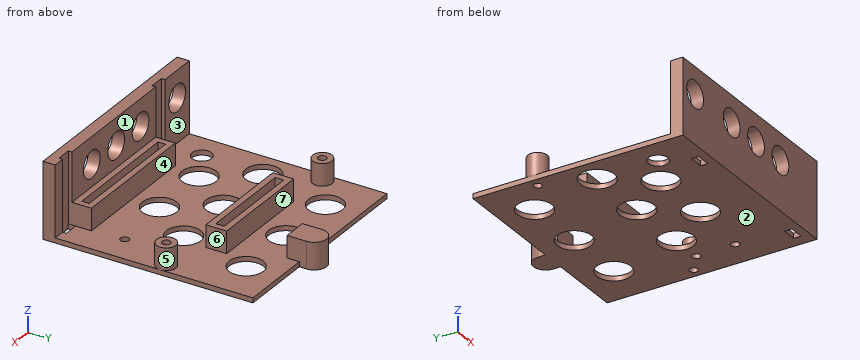
```python
from build123d import *

# Parameters (mm, degrees)
PAD_DEPTH       = 2
SKETCH001_W     = 50
SKETCH001_H     = 3
SKETCH001_W_2   = 44
SKETCH001_H_2   = 8.5
SKETCH001_W_3   = 39
SKETCH001_H_3   = 3.5
SKETCH001_R     = 4
PAD001_DEPTH    = 9
SKETCH003_R     = 1.75
SKETCH003_R_2   = 7
SKETCH003_R_3   = 4
SKETCH003_W     = 6
SKETCH003_H     = 3
POCKET_DEPTH    = 5
PAD002_DEPTH    = 20
SKETCH006_R     = 5.5
POCKET001_DEPTH = 5
SKETCH004_R     = 1.7
POCKET002_DEPTH = 11


with BuildPart() as part:
    # Sketch → Pad (new body)
    with BuildSketch(Plane.XY):
        with BuildLine():
            Line((0, 0), (0, 86))
            Line((0, 86), (47.5, 86))
            Line((47.5, 86), (47.5, 89))
            ThreePointArc((57.5, 89), (52.5, 94), (47.5, 89))
            Line((57.5, 89), (57.5, 86))
            Line((57.5, 86), (88, 86))
            Line((88, 86), (88, 0))
            Line((88, 0), (0, 0))
        make_face()
    extrude(amount=PAD_DEPTH)

    # Sketch001 → Pad001 (new body)
    with BuildSketch(Plane.XY.offset(2)):
        Polygon((0, 0), (0, 5), (15.9, 5), (15.9, 3.5), (22, 3.5), (22, 13), (77, 13), (77, 3.5), (83.1, 3.5), (83.1, 5), (88, 5), (88, 0), align=None)
        with Locations((49.5, 9)):
            Rectangle(SKETCH001_W, SKETCH001_H, mode=Mode.SUBTRACT)
        with Locations((44, 57.25)):
            Rectangle(SKETCH001_W_2, SKETCH001_H_2)
        with Locations((44, 57.25)):
            Rectangle(SKETCH001_W_3, SKETCH001_H_3, mode=Mode.SUBTRACT)
        with BuildLine():
            Line((47.5, 89), (47.5, 81))
            Line((47.5, 81), (57.5, 81))
            Line((57.5, 81), (57.5, 89))
            ThreePointArc((57.5, 89), (52.5, 94), (47.5, 89))
        make_face()
        with Locations((4, 62)):
            Circle(SKETCH001_R)
        with Locations((84, 48)):
            Circle(SKETCH001_R)
    extrude(amount=PAD001_DEPTH)

    # Sketch003 → Pocket (cut)
    with BuildSketch(Plane.XY.offset(2)):
        with Locations((76, 42)):
            Circle(SKETCH003_R)
        with Locations((76, 26)):
            Circle(SKETCH003_R)
        with Locations((37, 42)):
            Circle(SKETCH003_R_2)
        with Locations((24, 24)):
            Circle(SKETCH003_R_2)
        with Locations((63, 42)):
            Circle(SKETCH003_R_2)
        with Locations((50, 24)):
            Circle(SKETCH003_R_2)
        with Locations((70, 72)):
            Circle(SKETCH003_R_2)
        with Locations((44, 72)):
            Circle(SKETCH003_R_2)
        with Locations((18, 72)):
            Circle(SKETCH003_R_2)
        with Locations((11, 42)):
            Circle(SKETCH003_R_2)
        with Locations((11, 17)):
            Circle(SKETCH003_R_3)
        with Locations((80.1, 5)):
            Rectangle(SKETCH003_W, SKETCH003_H)
        with Locations((18.9, 5)):
            Rectangle(SKETCH003_W, SKETCH003_H)
    extrude(amount=-POCKET_DEPTH, mode=Mode.SUBTRACT)

    # Sketch005 → Pad002 (new body)
    with BuildSketch(Plane.XY.offset(11)):
        Polygon((0, 0), (0, 5), (15.9, 5), (15.9, 3.5), (22, 3.5), (22, 5), (77, 5), (77, 3.5), (83.1, 3.5), (83.1, 5), (88, 5), (88, 0), align=None)
    extrude(amount=PAD002_DEPTH)

    # Sketch006 → Pocket001 (cut)
    with BuildSketch(Plane.XZ):
        with Locations((8, 20)):
            Circle(SKETCH006_R)
        with Locations((32, 20)):
            Circle(SKETCH006_R)
        with Locations((48, 20)):
            Circle(SKETCH006_R)
        with Locations((64, 20)):
            Circle(SKETCH006_R)
    extrude(amount=-POCKET001_DEPTH, mode=Mode.SUBTRACT)

    # Sketch004 → Pocket002 (cut)
    with BuildSketch(Plane.XY.offset(11)):
        with Locations((4, 62)):
            Circle(SKETCH004_R)
        with Locations((84, 48)):
            Circle(SKETCH004_R)
    extrude(amount=-POCKET002_DEPTH, mode=Mode.SUBTRACT)


solid = part.part
```
Part model, mm, in its own coordinate system. Face numbers are marked on the shaded views. A direction names the side the tool comes from. Coordinates: 2 decimals unless noted, no trailing zeros. Write each loop counter-clockwise with the first axis right and the second up, starting at its lowest first coordinate (ties: lowest second). Pieces come first, ordered by that corner, then holes.
Item 1: Slice it at B-B (x = 34.5). Write the cut outline in (y, z).
Item 2: Slice it at A-A (z = 6.5). Count the separate pieces of the cut face and the enclosed holes in it, and give its area (3 significant figures).
Item 3: Pin check, flat tips, straight feed: pin 1 (17.5 mm diameter, centred on x = 8, z = 20, fed in from +Y); pin 2 (3 mm diameter, centred on x = 84, y = 48, fed in from -Z); pin 3 (9.5 mm diameter, centred on y = 57.5, z = 8, fed in from +X); pin 4 (0.6 mm diameter, centred on x = 21.5, z = 1.5, fed in from +Y). Stop position of each tip, or through.
Item 4: Slice it at D-D (y = 38). Write the cut outline in (x, z), and give its area (3 significant figures).
Item 5: Which spindle directions (+Z, -Z, +X, -X, +Y, -Y) get a long thin tool onto all of the face, cutting with end or side? Do the marked faces 4, 5, 6 and 7. Say none if no direction does.
Item 6: Mould opens along Y. For the marked faces 1, 2 and 3 say: released by +Y, released by -Y, zero draft, split by the parting line, or undercut.
Item 7: Slice it at C-C (y = 26). Write the cut outline in (x, z).
Item 8: Probe line 1 (Y direction, x = 32, z = 6); line 2 (Y direction, x = 84, z = 5.75); line 3 (Z direction, x = 32, y = 1). List the from-to ranges inside material, lowest first.
Results found:
1. outline: (0, 0) - (35.46, 0) - (35.46, 2) - (13, 2) - (13, 11) - (10.5, 11) - (10.5, 2) - (7.5, 2) - (7.5, 11) - (5, 11) - (5, 15.1) - (0, 15.1) - close; (0, 24.9) - (5, 24.9) - (5, 31) - (0, 31) - close; (48.54, 0) - (86, 0) - (86, 2) - (61.5, 2) - (61.5, 11) - (59, 11) - (59, 2) - (55.5, 2) - (55.5, 11) - (53, 11) - (53, 2) - (48.54, 2) - close
2. separate pieces: 5
2. enclosed holes: 4
2. area: 1,150 mm2
3. pin 1: stops at y = 5
3. pin 2: passes through
3. pin 3: stops at x = 66
3. pin 4: stops at y = 86
4. outline: (0, 0) - (5.26, 0) - (5.26, 2) - (0, 2) - close; (16.74, 0) - (31.26, 0) - (31.26, 2) - (16.74, 2) - close; (42.74, 0) - (57.26, 0) - (57.26, 2) - (42.74, 2) - close; (68.74, 0) - (88, 0) - (88, 2) - (68.74, 2) - close
4. area: 107 mm2
5. face 4: +Z, +X, -X
5. face 5: +Z
5. face 6: +Z, +X, +Y
5. face 7: +Z, +X
6. face 1: released by +Y
6. face 2: zero draft
6. face 3: undercut
7. outline: (0, 0) - (17.29, 0) - (17.29, 2) - (0, 2) - close; (30.71, 0) - (43.29, 0) - (43.29, 2) - (30.71, 2) - close; (56.71, 0) - (74.25, 0) - (74.25, 2) - (56.71, 2) - close; (77.75, 0) - (88, 0) - (88, 2) - (77.75, 2) - close
8. line 1: y = 0 to 7.5, 10.5 to 13, 53 to 55.5, 59 to 61.5
8. line 2: y = 0 to 5, 44 to 46.3, 49.7 to 52
8. line 3: z = 0 to 14.5, 25.5 to 31
